Build history of the part. All positions in model axes, mm. A direction names the side the tool comes from. Give positions to 0.01 mm unless a question says otherwise; leave off trailing zeros. Loops run counter-clockwise (first coordinate to the right, second up) from the corner with the lowest first, then second, coordinate; pieces in that order, holes last. Notation, with made-up numbers: M 2,-1.5 L 60,-1.5 A26 ccw 60,32.5 Z; hole C 34.25,33.25 d8. An arc over 180 degrees is marked long. Answer in a Markdown table with one row per item. Add a question column.
Autodesk Inventor part; units mm, degrees
ref_plane "YZ Plane" through (0, 0, 0) normal (1, 0, 0) x (0, 1, 0)
ref_plane "XZ Plane" through (0, 0, 0) normal (0, 1, 0) x (-1, 0, 0)
ref_plane "XY Plane" through (0, 0, 0) normal (0, 0, 1) x (1, 0, 0)
sketch "スケッチ1" plane through (0, 0, 0) normal (0, 0, 1) x (1, 0, 0)
  line L0 (108, 72.831817) -> (108, -27.637331) construction
  circle A0 centre (90, 27) radius 3
  circle A1 centre (104.07345, 2) radius 6.025
  circle A2 centre (90, 27) radius 1.5
  circle A3 centre (104.07345, 2) radius 1.5
  circle A4 centre (82.04031, 11.281864) radius 1.5
  circle A5 centre (82.5, -8) radius 3
  circle A6 centre (82.5, -8) radius 1.5
  arc A7 (66.645247, -5.64) -> (72.915941, -4.36) centre (69.780594, -5) ccw
  arc A8 (72.724551, 23.828571) -> (66.645247, -5.64) centre (104.07345, 2) ccw
  arc A9 (77.976723, 20.171429) -> (72.915941, -4.36) centre (104.07345, 2) ccw
  arc A10 (77.976723, 20.171429) -> (72.724551, 23.828571) centre (75.350637, 22) ccw
  circle A11 centre (137.322151, 20) radius 1.25
  circle A12 centre (133.5, -8) radius 3
  circle A13 centre (133.5, -8) radius 1.5
  circle A14 centre (146, 10) radius 1.5
  arc A15 (-6.089587, 13.373015) -> (73.990447, 1.93301) centre (42.288654, 66.020578) ccw construction
  line L1 (108, 72.831817) -> (108, -27.637331) construction
  arc A16 (142.009553, 1.93301) -> (222.089587, 13.373015) centre (173.711346, 66.020578) ccw construction
  arc A17 (142.29705, -19.072921) -> (142.660887, 27.253552) centre (125.709293, 4.222021) ccw
  arc A18 (136.80781, 35.127338) -> (180.06622, 10.718677) centre (180.861669, 62.665248) ccw
  circle A19 centre (137.322151, 20) radius 9.006449
  arc A20 (128.322651, 20.353731) -> (130.555913, -8.5765) centre (253.226204, 15.444317) ccw
  arc A21 (133.414591, -10.998784) -> (152.948723, -4.485529) centre (134.268683, 18.989056) ccw
  arc A22 (35.93378, 10.718677) -> (79.19219, 35.127338) centre (35.138331, 62.665248) ccw
  arc A23 (73.339113, 27.253552) -> (73.70295, -19.072921) centre (90.290707, 4.222021) ccw
  arc A24 (90.887703, 29.865656) -> (71.118535, 25.188537) centre (84.969685, 10.761283) ccw
  arc A25 (109.559222, 4.491371) -> (92.075879, 29.165808) centre (36.719095, -28.589074) ccw
  arc A26 (80.567193, -10.294397) -> (70.653319, -16.566942) centre (76.603177, -15) ccw
  circle A27 centre (76.603177, -15) radius 5 construction
  circle A28 centre (94, -11) radius 1.5
  circle A29 centre (94, -11) radius 3
  arc A30 (103.111347, -3.947687) -> (84.657245, -10.084777) centre (99.757959, -24.678215) ccw
  point P0 (0, 0)
  point P1 (0, 0)
  point P2 (153.490711, -2.560367)
  point P3 (70.420594, -8.135347)
  point P4 (68.814065, 23.104865)
  dimension "d0" = 2
  dimension "d1" = 30
  dimension "d2" = 125
  dimension "d3" = 80
  dimension "d4" = 20
  dimension "d5" = 6
  dimension "d6" = 21
extrude "押し出し1" add sketch "スケッチ1" along normal blind 3 contours A0 | A0 A25 A1 A30 A5 A26 A23 A22 A24 | A1 | A5
fillet "フィレット1" radius 5 1 edges at (68.8141, 23.1049, 1.5)
fillet "フィレット2" radius 2 1 edges at (70.6533, -16.5669, 1.5)
sketch "スケッチ2" plane through (0, 0, 0) normal (0, 0, -1) x (-1, 0, 0)
  circle A0 centre (-82.04031, 11.281864) radius 1.5
  arc A1 (-70.932275, -12.613165) -> (-67.494617, -13.044892) centre (-69.088898, -11.837303) ccw
  arc A2 (-67.494617, -13.044892) -> (-68.54743, 22.797215) centre (-90.290707, 4.222021) ccw
  arc A3 (-68.54743, 22.797215) -> (-69.082243, 23.334729) centre (-72.349055, 19.549502) ccw
  arc A4 (-71.118535, 25.188537) -> (-69.082243, 23.334729) centre (-35.138331, 62.665248) ccw
  arc A5 (-71.118535, 25.188537) -> (-90.887703, 29.865656) centre (-84.969685, 10.761283) ccw
  arc A6 (-90.887703, 29.865656) -> (-92.075879, 29.165808) centre (-90, 27) ccw
  arc A7 (-92.075879, 29.165808) -> (-109.559222, 4.491371) centre (-36.719095, -28.589074) ccw
  arc A8 (-109.559222, 4.491371) -> (-103.111347, -3.947687) centre (-104.07345, 2) ccw
  arc A9 (-84.657245, -10.084777) -> (-103.111347, -3.947687) centre (-99.757959, -24.678215) ccw
  arc A10 (-84.657245, -10.084777) -> (-80.567193, -10.294397) centre (-82.5, -8) ccw
  arc A11 (-70.932275, -12.613165) -> (-80.567193, -10.294397) centre (-76.603177, -15) ccw
  circle A12 centre (-82.5, -8) radius 1.5
  circle A13 centre (-104.07345, 2) radius 1.5
  circle A14 centre (-90, 27) radius 1.5
  circle A15 centre (-82.04031, 11.281864) radius 1.5
  arc A16 (-72.724551, 23.828571) -> (-77.976723, 20.171429) centre (-75.350637, 22) ccw
  arc A17 (-66.645247, -5.64) -> (-72.724551, 23.828571) centre (-104.07345, 2) ccw
  arc A18 (-72.915941, -4.36) -> (-66.645247, -5.64) centre (-69.780594, -5) ccw
  arc A19 (-72.915941, -4.36) -> (-77.976723, 20.171429) centre (-104.07345, 2) ccw
  circle A20 centre (-90, 27) radius 3.1
  circle A21 centre (-82.04031, 11.281864) radius 3.1
  circle A22 centre (-104.07345, 2) radius 3.1
  circle A23 centre (-82.5, -8) radius 3.1
  arc A24 (-86.256515, -9.37426) -> (-87.720107, -7.470946) centre (-90.013031, -10.748521) ccw
  arc A25 (-86.256515, -9.37426) -> (-79.334786, -10.445694) centre (-82.5, -8) ccw
  arc A26 (-75.363887, -8.973369) -> (-79.334786, -10.445694) centre (-76.169572, -12.891388) ccw
  arc A27 (-70.932275, -12.613165) -> (-80.567193, -10.294397) centre (-76.603177, -15) ccw
  arc A28 (-94.623726, 26.61105) -> (-93.882942, 27.960603) centre (-96.795149, 28.681055) ccw
  arc A29 (-88.670242, 30.772498) -> (-93.882942, 27.960603) centre (-90, 27) ccw
  arc A30 (-88.670242, 30.772498) -> (-87.320327, 30.622665) centre (-87.672923, 33.601872) ccw
  point P0 (0, 0)
  dimension "d11" = 6.2
  dimension "d12" = 6.2
  dimension "d13" = 6.2
  dimension "d14" = 6.2
  dimension "d15" = 4
  dimension "d16" = 4
  dimension "d17" = 4
  dimension "d18" = 4
  dimension "d19" = 3
  dimension "d20" = 3
extrude "押し出し2" add sketch "スケッチ2" against normal up to surface (3 mm away) contours A26 A25 A24 A9 A23 A11 | A23 A9 A10 A11 | A5 A20 A7 A28 A29 A30 | A5 A6 A7 A20 picked at (-81.994217, -10.979131) picked at (-91.467973, 29.678904)
extrude "押し出し3" cut sketch "スケッチ2" against normal blind 1 contours A23 A9 A10 A11 | A11 A10 A9 A23 | A20 A7 A6 A5 | A5 A6 A7 A20 | A12 | A14 | A21 | A22
sketch "スケッチ4" plane through (0, 0, 3) normal (0, 0, 1) x (1, 0, 0)
  arc A0 (67.494617, -13.044892) -> (70.932275, -12.613165) centre (69.088898, -11.837303) ccw
  arc A1 (75.363887, -8.973369) -> (70.932275, -12.613165) centre (76.603177, -15) ccw
  arc A2 (79.334786, -10.445694) -> (75.363887, -8.973369) centre (76.169572, -12.891388) ccw
  arc A3 (79.334786, -10.445694) -> (86.256515, -9.37426) centre (82.5, -8) ccw
  arc A4 (87.720107, -7.470946) -> (86.256515, -9.37426) centre (90.013031, -10.748521) ccw
  arc A5 (103.111347, -3.947687) -> (87.720107, -7.470946) centre (99.757959, -24.678215) ccw
  arc A6 (103.111347, -3.947687) -> (109.559222, 4.491371) centre (104.07345, 2) ccw
  arc A7 (109.559222, 4.491371) -> (94.623726, 26.61105) centre (36.719095, -28.589074) ccw
  arc A8 (93.882942, 27.960603) -> (94.623726, 26.61105) centre (96.795149, 28.681055) ccw
  arc A9 (93.882942, 27.960603) -> (88.670242, 30.772498) centre (90, 27) ccw
  arc A10 (87.320327, 30.622665) -> (88.670242, 30.772498) centre (87.672923, 33.601872) ccw
  arc A11 (87.320327, 30.622665) -> (71.118535, 25.188537) centre (84.969685, 10.761283) ccw
  arc A12 (69.082243, 23.334729) -> (71.118535, 25.188537) centre (35.138331, 62.665248) ccw
  arc A13 (69.082243, 23.334729) -> (68.54743, 22.797215) centre (72.349055, 19.549502) ccw
  arc A14 (68.54743, 22.797215) -> (67.494617, -13.044892) centre (90.290707, 4.222021) ccw
  circle A15 centre (82.5, -8) radius 1.5
  circle A16 centre (104.07345, 2) radius 1.5
  circle A17 centre (90, 27) radius 1.5
  circle A18 centre (82.04031, 11.281864) radius 1.5
  arc A19 (77.976723, 20.171429) -> (72.724551, 23.828571) centre (75.350637, 22) ccw
  arc A20 (77.976723, 20.171429) -> (72.915941, -4.36) centre (104.07345, 2) ccw
  arc A21 (66.645247, -5.64) -> (72.915941, -4.36) centre (69.780594, -5) ccw
  arc A22 (72.724551, 23.828571) -> (66.645247, -5.64) centre (104.07345, 2) ccw
  arc A23 (70.112674, 24.248139) -> (65.061877, -9.243272) centre (104.07345, 2) ccw
  arc A24 (72.724551, 23.828571) -> (66.645247, -5.64) centre (104.07345, 2) ccw
  arc A25 (77.522944, 29.323235) -> (67.556607, 19.743566) centre (85.545451, 11.002771) ccw
  point P0 (0, 0)
  dimension "d28" = 20
sketch "スケッチ4 outline for 押し出し4" plane through (0, 0, 3) normal (0, 0, 1) x (1, 0, 0)
  arc A0 (69.082243, 23.334729) -> (68.54743, 22.797215) centre (72.349055, 19.549502) ccw
  arc A1 (68.54743, 22.797215) -> (65.061877, -9.243272) centre (90.290707, 4.222021) ccw
  arc A2 (65.061877, -9.243272) -> (67.556607, 19.743566) centre (104.07345, 2) cw
  arc A3 (67.556607, 19.743566) -> (77.522944, 29.323235) centre (85.545451, 11.002771) cw
  arc A4 (77.522944, 29.323235) -> (71.118535, 25.188537) centre (84.969685, 10.761283) ccw
  arc A5 (71.118535, 25.188537) -> (69.082243, 23.334729) centre (35.138331, 62.665248) cw
extrude "押し出し4" cut sketch "スケッチ4 outline for 押し出し4" against normal blind 10
fillet "フィレット3" radius 2 1 edges at (65.0619, -9.2433, 1.5)
properties part number "アンノーン前" material "アルミニウム 2014-T4"
(1) Slice it at C-C, the plane y = 15. Give the cut face in (x, z), then the cut area to 3 significant figures.
(2) Slice it at D-D, the plane x = 90. Give the cut face in (y, z), then the cut area to 3 significant figures.
(3) Slice it at A-A, the plane y = 2. Give the cut face in (x, z).
(4) Wall check: line 1 (X direction, y = 4.5, z = 0.75); line 2 (Y direction, x = 81, z = 0.35); line 3 (X direction, y = 11.5, z = 0.5). Give the ranges that are in metal, low to high.
(5) Pin check, flat tips, straight feed: pin 1 (3 mm diameter, centred on x = 78, y = -4, fed in from -Z); pin 2 (3 mm diameter, centred on x = 104.5, y = 1.5, fed in from -Z); pin 3 (1 mm diameter, centred on x = 73, z = 0.5, fed in from +Y); pin 4 (1 mm diameter, centred on x = 84, z = 0.5, fed in from +Y). Stop position of each tip, or through.
(6) Pull direction X, two halves, no side cores. Call faces 5 (the cylindrical face through (102.92, 16.33, 1.48)), 6 (the cylindrical face through (85.137, 11.418, 0.493)), 7 (the flat face through (86, 9, 3)): +X half, -X half, draft (parallel to the pull), parting line (faces both ways), or undercut.
(7) Tool access for faces 1 (the cylindrical face through (66.28, -11.31, 1.48)), 2 (the cylindrical face through (101.117, 2.931, 0.493)), 3 (the cylindrical face through (72.893, 8.248, 1.479)), 4 (the cylindrical face through (72.67, -10.27, 1.48)): list every direction of +Z, -Z, +X, -X, +Y, -Y with a clear straight run to the whole face (end or side of a thin tool).
(8) Slice it at B-B, the plane x = 82.5. Give the cut face in (y, z).
Solution:
| question | item | result |
|---|---|---|
| 1 | outline | M 65.61,0 L 68.15,0 L 68.15,3 L 65.61,3 Z; M 75.05,0 L 103.8,0 L 103.8,3 L 75.05,3 Z |
| 1 | area | 93.9 mm^2 |
| 2 | outline | M -6.08,0 L 23.9,0 L 23.9,1 L 25.5,1 L 25.5,3 L -6.08,3 Z; M 28.5,1 L 30.1,1 L 30.1,0 L 31,0 L 31,3 L 28.5,3 Z |
| 2 | area | 99.0 mm^2 |
| 3 | outline | M 63.47,0 L 65.87,0 L 65.87,3 L 63.47,3 Z; M 72.27,0 L 100.97,0 L 100.97,1 L 102.57,1 L 102.57,3 L 72.27,3 Z; M 105.57,1 L 107.17,1 L 107.17,0 L 110.1,0 L 110.1,3 L 105.57,3 Z |
| 4 | line 1 | 63.55 to 65.96, 72.37 to 102.24, 105.91 to 109.56 |
| 4 | line 2 | -11.71 to -10.71, -5.29 to 8.36, 14.2 to 30.36 |
| 4 | line 3 | 64.6 to 67.07, 73.73 to 78.95, 85.13 to 105.95 |
| 5 | pin 1 | z = 0 |
| 5 | pin 2 | z = 1 |
| 5 | pin 3 | y = 26.97 |
| 5 | pin 4 | y = 30.76 |
| 6 | face 5 | +X half |
| 6 | face 6 | undercut |
| 6 | face 7 | draft |
| 7 | face 1 | +Z, -Z, -X, -Y |
| 7 | face 2 | -Z |
| 7 | face 3 | +Z, -Z |
| 7 | face 4 | +Z, -Z, -Y |
| 8 | outline | M -12,0 L -11.1,0 L -11.1,1 L -9.5,1 L -9.5,3 L -12,3 Z; M -6.5,1 L -4.9,1 L -4.9,0 L 8.22,0 L 8.22,1 L 9.85,1 L 9.85,3 L -6.5,3 Z; M 12.71,1 L 14.35,1 L 14.35,0 L 30.61,0 L 30.61,3 L 12.71,3 Z |
